Read the model definition and answer for the solid it produces. Units are mm, in the model's axes. A direction names the side the tool comes from. Coordinates: 2 decimals unless noted, no trailing zeros. Loops run counter-clockwise (first coordinate to the right, second up) from the corner with the lowest first, then second, coordinate; pieces in that order, holes last.
from build123d import *

# Parameters (mm, degrees)
BOSS_EXTRUDE1_DEPTH   = 3.000000096
SKETCH2_R             = 3.175
CUT_EXTRUDE1_DEPTH    = 4.000000096
SKETCH3_W             = 2.54
SKETCH3_H             = 0.635
CUT_EXTRUDE2_DEPTH    = 4.000000096
BOSS_EXTRUDE2_DEPTH   = 2.206999904
F_6_32_TAPPED_HOLE1_D = 2.7051


with BuildPart() as part:
    # Sketch1 → Boss-Extrude1 (new body)
    with BuildSketch(Plane.XY):
        with BuildLine():
            Line((27.218819563, 62.393373411), (22.357699804, 50.65759216))
            ThreePointArc((22.357699804, 50.65759216), (28.61353693, 47.405947816), (34.405475059, 43.38573118))
            Line((34.405475059, 43.38573118), (8.696654013, 17.676910134))
            Line((8.696654013, 17.676910134), (7.228954972, 14.133571205))
            ThreePointArc((7.228954972, 14.133571205), (14.666587579, 6.075099489), (15.105587123, -4.88230096))
            Line((15.105587123, -4.88230096), (18.648926052, -6.35))
            Line((18.648926052, -6.35), (101.401368334, -6.35))
            ThreePointArc((101.401368334, -6.35), (93.866160503, 38.880636728), (67.21146711, 76.191723231))
            Line((67.21146711, 76.191723231), (43.43415954, 52.414415661))
            ThreePointArc((43.43415954, 52.414415661), (35.677104191, 57.973626939), (27.218819563, 62.393373411))
        make_face()
        with BuildLine():
            Line((88.672924278, 6.35), (27.86051193, 6.35))
            ThreePointArc((27.86051193, 6.35), (26.399857642, 10.93517908), (24.190484974, 15.210228852))
            Line((24.190484974, 15.210228852), (67.191354125, 58.211098004))
            ThreePointArc((67.191354125, 58.211098004), (82.13289044, 34.020557137), (88.672924278, 6.35))
        make_face(mode=Mode.SUBTRACT)
    extrude(amount=BOSS_EXTRUDE1_DEPTH)

    # Sketch2 → Cut-Extrude1 (cut, through all)
    with BuildSketch(Plane.XY.offset(3.000000096)):
        with Locations((22.225, 0)):
            Circle(SKETCH2_R)
        with Locations((36.195, 0)):
            Circle(SKETCH2_R)
        with Locations((61.722, 0)):
            Circle(SKETCH2_R)
        with Locations((75.692, 0)):
            Circle(SKETCH2_R)
        with Locations((95.25, 0)):
            Circle(SKETCH2_R)
        with Locations((15.715448212, 15.715448212)):
            Circle(SKETCH2_R)
        with Locations((25.593729945, 25.593729945)):
            Circle(SKETCH2_R)
        with Locations((43.644044748, 43.644044748)):
            Circle(SKETCH2_R)
        with Locations((53.522326482, 53.522326482)):
            Circle(SKETCH2_R)
        with Locations((92.004434954, 24.652514046)):
            Circle(SKETCH2_R)
        with Locations((82.48891971, 47.625)):
            Circle(SKETCH2_R)
        with Locations((67.351920908, 67.351920908)):
            Circle(SKETCH2_R)
    extrude(amount=-CUT_EXTRUDE1_DEPTH, mode=Mode.SUBTRACT)

    # Sketch3 → Cut-Extrude2 (cut, through all)
    with BuildSketch(Plane.XY.offset(3.000000096)):
        Polygon((15.266435406, 24.246691527), (17.06248663, 26.042742751), (17.511499436, 25.593729945), (15.715448212, 23.797678721), align=None)
        Polygon((43.43415954, 52.414415661), (44.991083167, 53.971339288), (53.971339288, 44.991083167), (52.414415661, 43.43415954), align=None)
        with Locations((29.21, -6.0325)):
            Rectangle(SKETCH3_W, SKETCH3_H)
        with Locations((68.707, -6.0325)):
            Rectangle(SKETCH3_W, SKETCH3_H)
        Polygon((29.230733674, 38.210989795), (31.026784898, 40.007041019), (31.475797704, 39.558028213), (29.67974648, 37.761976989), align=None)
        Polygon((56.845021246, 65.825277367), (55.048970022, 64.029226143), (55.497982828, 63.580213337), (57.294034052, 65.376264561), align=None)
        with Locations((48.9585, -6.0325)):
            Rectangle(SKETCH3_W, SKETCH3_H)
        with Locations((85.471, -6.0325)):
            Rectangle(SKETCH3_W, SKETCH3_H)
        Polygon((99.935462164, 14.437711971), (100.266998693, 11.919442024), (101.526133667, 12.085210288), (101.194597138, 14.603480236), align=None)
        Polygon((93.765504959, 37.464305742), (94.938831965, 37.950313702), (93.966816047, 40.296967714), (92.793489041, 39.810959755), align=None)
        Polygon((79.327792988, 62.471156422), (80.874047017, 60.456038938), (81.88160576, 61.229165953), (80.33535173, 63.244283437), align=None)
        Polygon((13.593916116, 7.005422516), (14.565932035, 4.658768503), (15.739259041, 5.144776462), (14.767243123, 7.491430475), align=None)
    extrude(amount=-CUT_EXTRUDE2_DEPTH, mode=Mode.SUBTRACT)

    # Sketch4 → Boss-Extrude2 (add)
    with BuildSketch(Plane.XY.offset(3.000000096)):
        with BuildLine():
            Line((22.357699804, 50.65759216), (27.218819563, 62.393373411))
            ThreePointArc((27.218819563, 62.393373411), (35.13186657, 58.305652688), (42.443492672, 53.219800017))
            Line((42.443492672, 53.219800017), (33.393246405, 44.169553751))
            ThreePointArc((33.393246405, 44.169553751), (28.063600293, 47.73355971), (22.357699804, 50.65759216))
        make_face()
    extrude(amount=BOSS_EXTRUDE2_DEPTH)

    # #6-32 Tapped Hole1 (through all)
    with Locations(Plane(origin=(0, 0, 0), x_dir=(-1, 0, 0), z_dir=(0, 0, -1))):
        with Locations((-30.861, 53.452819972)):
            Hole(F_6_32_TAPPED_HOLE1_D / 2)


solid = part.part
Q1. A cutting plane is placed at A-A (y = 0). Give the vertices of the cut face in (x, z) (3 decimals).
Findings below:
outline: (15.875, 0) - (19.05, 0) - (19.05, 3) - (15.875, 3) - close; (25.4, 0) - (33.02, 0) - (33.02, 3) - (25.4, 3) - close; (39.37, 0) - (58.547, 0) - (58.547, 3) - (39.37, 3) - close; (64.897, 0) - (72.517, 0) - (72.517, 3) - (64.897, 3) - close; (78.867, 0) - (92.075, 0) - (92.075, 3) - (78.867, 3) - close; (98.425, 0) - (101.6, 0) - (101.6, 3) - (98.425, 3) - close
Q2. Determine the mould class of faces 6 (the face through (88.072, 50.654, 1.479)), 7 (the face through (15.875, 0.069, 1.479)), 8 (the face through (26.426, 10.873, 1.479)) for opening direction X: +X half, -X half, draft (parallel to the pull), parting line (faces both ways), or undercut.
Findings below:
face 6: +X half
face 7: -X half
face 8: undercut
Q3. Flat-ended cylindrical pins translate along their axes: pin 1 Ø1.5 at (x, y) = (43.5, 34) entering from -Z; pin 2 Ø7.5 at (x, y) = (75.692, 0) entering from +Z; pin 3 Ø0.8 at (x, z) = (85.5, 2) entering from -Y (3 decimals); pin 4 Ø4 at (x, y) = (22.225, 0) entering from +Z. Find the tip coordinate at first contact, or state that the pin passes through.
Findings below:
pin 1: stops at z = 0
pin 2: stops at z = 3
pin 3: stops at y = -5.715
pin 4: passes through
Q4. Which of the six approach directions +Z, -Z, +X, -X, +Y, -Y give full straight-line access (tool end or side, diameter ignored) to faces 1 (the face through (43.7, 35.1, 0)), 2 (the face through (29, -5.715, 2)), 3 (the face through (62.1, 71.08, 1.48)), 4 (the face through (23.23, 32.21, 1.48)), 5 (the face through (60.49, 51.51, 1.48))?
Findings below:
face 1: -Z, +X, -X, +Y, -Y
face 2: +Z, -Z, -Y
face 3: +Z, -Z, -X, +Y
face 4: +Z, -Z, -X
face 5: +Z, -Z
Q5. A cutting plane is placed at B-B (x = 75.5). Give the vertices of the cut face in (y, z), then the cut area to 3 significant figures.
Findings below:
outline: (-6.35, 0) - (-3.17, 0) - (-3.17, 3) - (-6.35, 3) - close; (3.17, 0) - (6.35, 0) - (6.35, 3) - (3.17, 3) - close; (46.94, 0) - (67.99, 0) - (67.99, 3) - (46.94, 3) - close
area: 82.2 mm2
Q6. A cutting plane is placed at C-C (z = 4.25). Give the vertices of the cut face in (x, y), then the cut area to 3 significant figures.
Findings below:
outline: (22.36, 50.66) arc R55.37 cw to (33.39, 44.17) - (42.44, 53.22) arc R68.07 ccw to (27.22, 62.39) - close; hole circle Ø2.71 at (30.86, 53.45)
area: 189 mm2
Q7. Straight lines are drawn through the part: probe 1 along Y at (x, z) = (80.5, 2.65); probe 2 along X at (y, z) = (23, 0.5); probe 3 along Y at (x, z) = (66, 2.35). For each, find the intervals that lie inside material, in ascending order.
Findings below:
probe 1: y = -6.35 to 6.35, 37.72 to 45.15, 50.1 to 60.94
probe 2: x = 14.02 to 23.76, 27.42 to 31.98, 85.87 to 89.29, 94.72 to 98.96
probe 3: y = -6.35 to 6.35, 57.02 to 64.48, 70.22 to 74.98
